Model file for the job. Use its own axes, mm. Give positions to 0.01 mm unless a question says otherwise; leave off trailing zeros. Loops run counter-clockwise (first coordinate to the right, second up) from the corner with the lowest first, then second, coordinate; pieces in that order, holes last. Notation, with made-up numbers: M -17,40.5 L 22,40.5 A21 cw 22,53.5 Z; hole C 69,-6.75 d6. An arc over 180 degrees is marked long. Answer in a Markdown table with one row per item.
Solid Edge part; units mm, degrees
sketch "Sketch1" plane through (0, 0, 0) normal (0, -1, 0) x (1, 0, 0)
  line L0 (8.5, 0) -> (8.5, 66.5)
  line L1 (-8.5, 66.5) -> (-8.5, 0)
  arc A0 (-8.5, 66.5) -> (8.5, 66.5) centre (0, 66.5) cw
  arc A1 (8.5, 0) -> (-8.5, 0) centre (0, 0) cw
  circle A2 centre (0, 66.5) radius 2.5
  circle A3 centre (0, 0) radius 2.5
extrude "Protrusion1" add sketch "Sketch1" against normal blind 1
(1) Mould opens along Z. For faces 1 (the cylindrical face through (-0.54, 0.49, 64.06)), 2 (the flat face through (0, 0, 34)), 3 (the cylindrical face through (-0.187, 0.493, -8.498)) say: pulls with the +Z half, pulls with the -Z half, needs draft (parallel to the pull), parting line crosses it, or undercut.
Established:
| item | result |
|---|---|
| face 1 | undercut |
| face 2 | needs draft |
| face 3 | pulls with the -Z half |
(2) Saw through at B-B, the plane y = 0.5. Give the cut face in (x, z), and give its area (3 significant figures).
Established:
| item | result |
|---|---|
| outline | M -8.5,0 A8.5 ccw 8.5,0 L 8.5,66.5 A8.5 ccw -8.5,66.5 Z; hole C 0,0 d5; hole C 0,66.5 d5 |
| area | 1,320 mm2 |
(3) Saw through at C-C, the plane x = 6.25. Give the cut face in (y, z).
Established:
| item | result |
|---|---|
| outline | M 0,-5.76 L 1,-5.76 L 1,72.26 L 0,72.26 Z |
(4) Saw through at A-A, the plane x = 0. Give the cut face in (y, z).
Established:
| item | result |
|---|---|
| outline | M 0,-8.5 L 1,-8.5 L 1,-2.5 L 0,-2.5 Z; M 0,2.5 L 1,2.5 L 1,64 L 0,64 Z; M 0,69 L 1,69 L 1,75 L 0,75 Z |
(5) Wall check: L1, parallel to Z at x = 0, y = 0.3; L2, parallel to Z at x = 2, y = 0.7; L3, parallel to X at y = 0.5, z = 65.5. Give the ranges that are in metal, low to high.
Established:
| item | result |
|---|---|
| L1 | z = -8.5 to -2.5, 2.5 to 64, 69 to 75 |
| L2 | z = -8.26 to -1.5, 1.5 to 65, 68 to 74.76 |
| L3 | x = -8.5 to -2.29, 2.29 to 8.5 |
